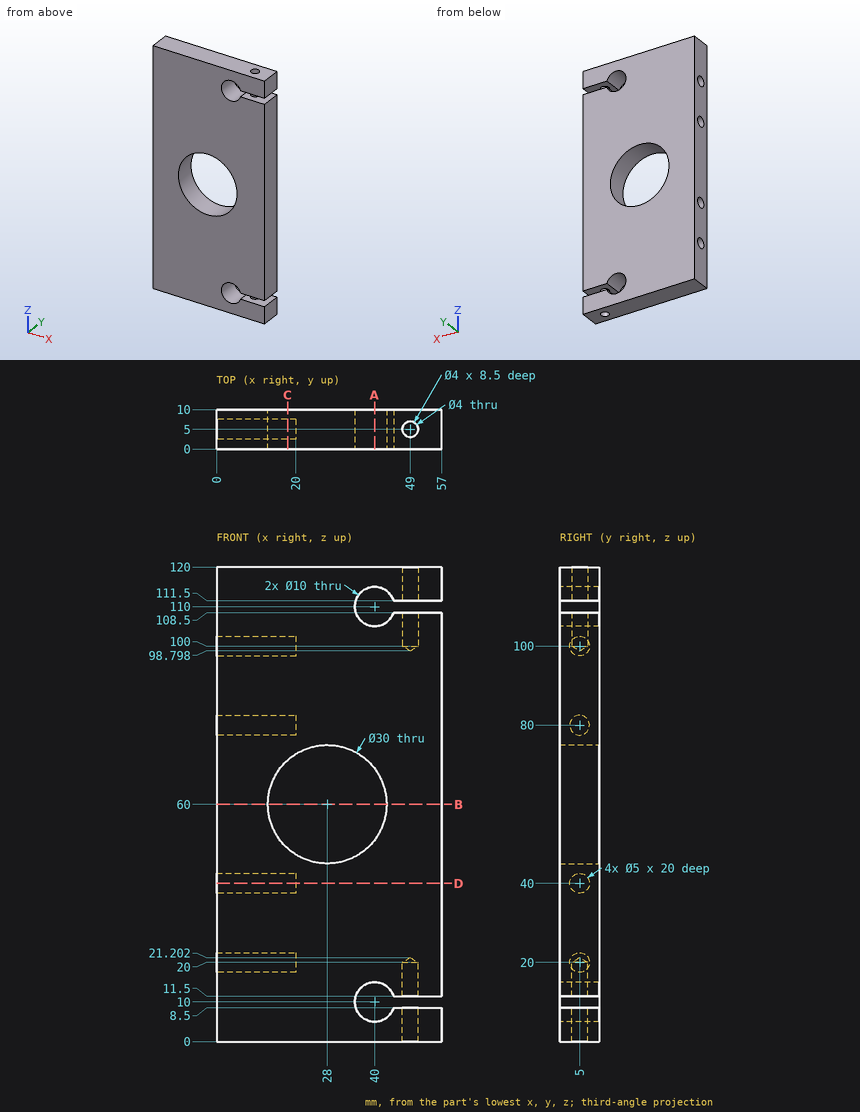
The figure shows three views and two pictorial views of one solid part (mm, origin at its lowest corner). Answer the questions. Coordinates: 2 decimals unless noted, no trailing zeros. Write each loop counter-clockwise with the first axis right and the second up, starting at its lowest first coordinate (ties: lowest second). Pieces come first, ordered by that corner, then holes. Notation, with made-up numbers: M 62.5,71 L 117.5,71 A28 cw 117.5,97 Z; hole C 53,-32 d8. An arc over 180 degrees is marked long. Answer as CSV lines item,"result". Start each with the question number.
Item 1: Section B-B on z = 60 is taken. Write down the section's boundary in (x, y).
Item 2: Section A-A on x = 40 is taken. Write down the section's boundary in (y, z), and give its area (3 significant figures).
Item 3: Section C-C on x = 18 is taken. Write down the section's boundary in (y, z), and give its area (3 significant figures).
Item 4: Section D-D on z = 40 is taken. Write down the section's boundary in (x, y).
Item 5: Consider L1, parallel to Z at x = 6.5, y = 5; L2, parallel to Z at x = 50, y = 2.25; L3, parallel to Y at x = 49, z = 5.5. Determine where each line is inside the solid, lowest interval first.
Item 6: Flat-ended cylindrical pins translate along their axes: P1, Ø5, axis at x = 49, y = 5, coming from the +Z side; P2, Ø3, axis at y = 5, z = 100, coming from the -X side; P3, Ø3, axis at x = 49, y = 5, coming from the +Z side. Find the tip coordinate at first contact, or state that the pin passes through.
Checks:
1,outline,"M 0,0 L 13,0 L 13,10 L 0,10 Z; M 43,0 L 57,0 L 57,10 L 43,10 Z"
2,outline,"M 0,0 L 10,0 L 10,5 L 0,5 Z; M 0,15 L 10,15 L 10,51 L 0,51 Z; M 0,69 L 10,69 L 10,105 L 0,105 Z; M 0,115 L 10,115 L 10,120 L 0,120 Z"
2,area,"820 mm²"
3,outline,"M 0,0 L 10,0 L 10,48.82 L 0,48.82 Z; M 0,71.18 L 10,71.18 L 10,120 L 0,120 Z; hole C 5,20 d5; hole C 5,40 d5; hole C 5,80 d5; hole C 5,100 d5"
3,area,"898 mm²"
4,outline,"M 0,0 L 57,0 L 57,10 L 0,10 L 0,7.5 L 20,7.5 L 20,2.5 L 0,2.5 Z"
5,L1,"z = 0 to 17.5, 22.5 to 37.5, 42.5 to 77.5, 82.5 to 97.5, 102.5 to 120"
5,L2,"z = 0 to 8.5, 11.5 to 108.5, 111.5 to 120"
5,L3,"y = 0 to 3, 7 to 10"
6,P1,"stops at z = 120"
6,P2,"stops at x = 20"
6,P3,"stops at z = 99.7"
